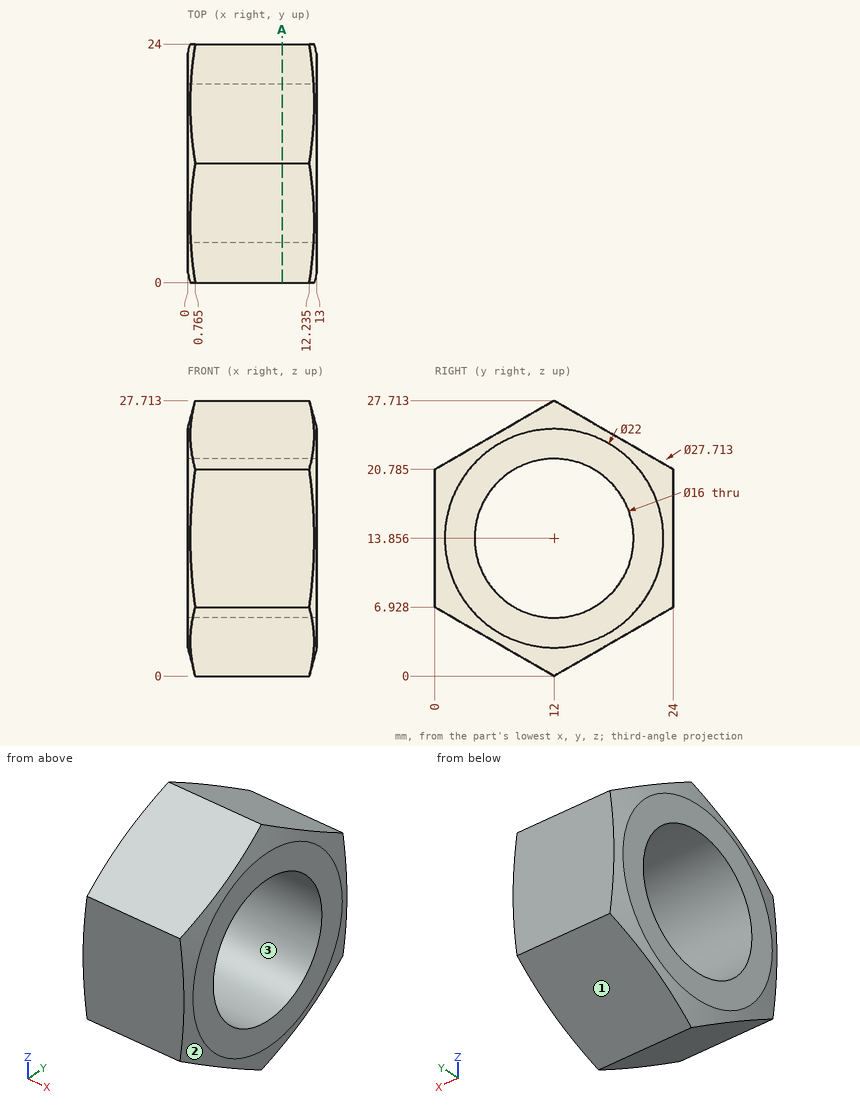
The figure shows three views and two pictorial views of one solid part (mm, origin at its lowest corner). Answer the questions. Coordinates: 2 decimals unless noted, no trailing zeros. Write each loop counter-clockwise with the first axis right and the second up, starting at its lowest first coordinate (ties: lowest second). Pieces come first, ordered by that corner, then holes.
1. Flat-ended cylindrical pins translate along their axes: pin 1 (5 mm diameter, centred on y = 14.5, z = 6, fed in from -X); pin 2 (1.5 mm diameter, centred on y = 21.5, z = 5.5, fed in from -X); pin 3 (3 mm diameter, centred on x = 5.5, y = 6.5, fed in from +Z). Find the tip coordinate at first contact, or state that the pin passes through.
Results list:
pin 1: stops at x = 0
pin 2: stops at x = 0.24
pin 3: stops at z = 25.4
2. The part is cut by section A-A, the plane x = 9.5. Write down the section's boundary in (y, z) (1 decimal).
Results list:
outline: (0, 6.9) - (12, 0) - (24, 6.9) - (24, 20.8) - (12, 27.7) - (0, 20.8) - close; hole circle Ø16 at (12, 13.9)
3. For a pull along Z with two mould halves and no side action, classify the marked faces 1, 2 and 3 as +Z half, -Z half, draft (parallel to the pull), parting line (faces both ways), or undercut.
Results list:
face 1: -Z half
face 2: parting line
face 3: undercut
4. Consider line 1 along Y through (x, z) = (11.25, 14); line 2 along Y through (x, z) = (3, 10.75); line 3 along Z through (x, y) = (9, 7.5) (1 decimal). Determine where each line is inside the solid, lowest interval first.
Results list:
line 1: y = 0 to 4, 20 to 24
line 2: y = 0 to 4.63, 19.37 to 24
line 3: z = 2.6 to 7.2, 20.5 to 25.1
